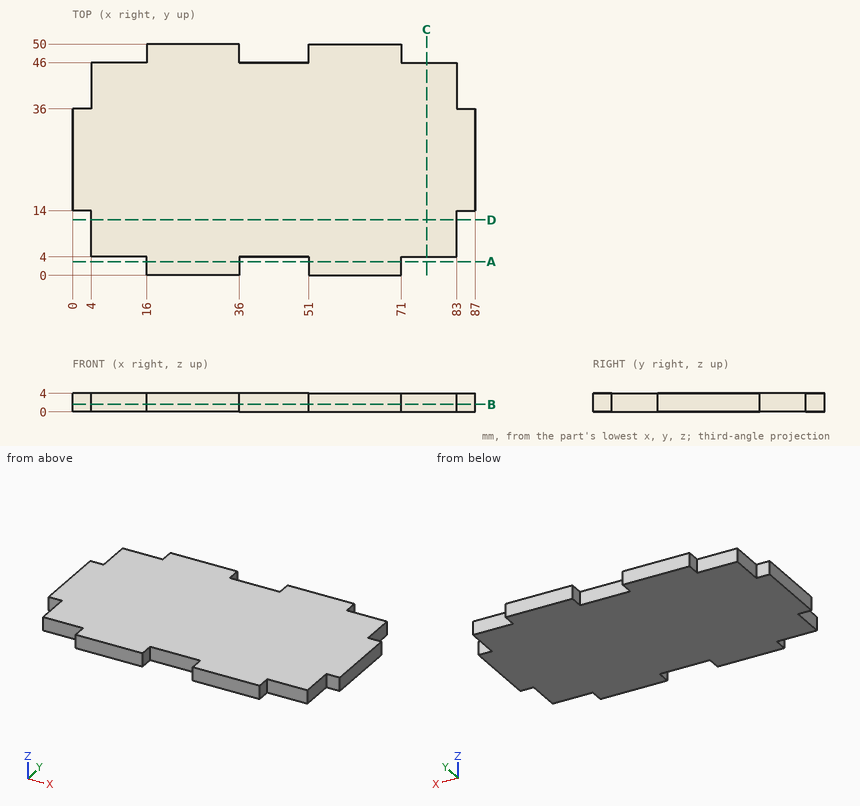
The drawing under review shows one solid part. Ordinate dimensions are in mm from its lowest x, y, z. Give positions to 0.01 mm unless a question says otherwise; leave off trailing zeros. Order: outer loops, then holes, each group sorted by start corner. A loop starts at its lowest first (then second) coordinate and runs counter-clockwise, first axis right, second up. Notation, with made-up numbers: (71.25, -17) -> (114.25, -17) arc R16 cw to (114.25, 12) -> close; hole circle Ø3 at (-1.5, 56). An arc over 180 degrees is marked (long way). Write item = value, one per line.
1) We need section C-C, the plane x = 76.5. Give the boundary of the cut face in (y, z), and give its area (3 significant figures).
Findings:
outline = (4, 0) -> (46, 0) -> (46, 4) -> (4, 4) -> close
area = 168 mm^2
2) We need section A-A, the plane y = 3. Give the boundary of the cut face in (x, z).
Findings:
outline = (16, 0) -> (36, 0) -> (36, 4) -> (16, 4) -> close; (51, 0) -> (71, 0) -> (71, 4) -> (51, 4) -> close
3) Insertion check: pin 1 (2 mm diameter, centred on x = 1, z = 2.5, fed in from -Y); pin 2 (1.2 mm diameter, centred on x = 46, z = 2.5, fed in from -Y); pin 3 (2 mm diameter, centred on y = 47.5, z = 2.5, fed in from -X). Each pin has a flat end and moves straight along its axis. Give the tip position at first contact, or say it passes through.
Findings:
pin_1 = 14
pin_2 = 4
pin_3 = 16
4) We need section B-B, the plane z = 1.6. Give the boundary of the cut face in (x, y), and give its area (3 significant figures).
Findings:
outline = (0, 14) -> (4, 14) -> (4, 4) -> (16, 4) -> (16, 0) -> (36, 0) -> (36, 4) -> (51, 4) -> (51, 0) -> (71, 0) -> (71, 4) -> (83, 4) -> (83, 14) -> (87, 14) -> (87, 36) -> (83, 36) -> (83, 46) -> (71, 46) -> (71, 50) -> (51, 50) -> (51, 46) -> (36, 46) -> (36, 50) -> (16, 50) -> (16, 46) -> (4, 46) -> (4, 36) -> (0, 36) -> close
area = 3,810 mm^2
5) To check wall thickness, follow L1, parallel to Y at x = 43.5, z = 3.85; L2, parallel to X at y = 38.5, z = 1.05. State the ranges of each line that lie inside material, in increasing order. Write a range as from..to.
Findings:
L1 = 4..46
L2 = 4..83
6) We need section D-D, the plane y = 12. Give the boundary of the cut face in (x, z).
Findings:
outline = (4, 0) -> (83, 0) -> (83, 4) -> (4, 4) -> close
